Autodesk Inventor part; units mm, degrees
ref_plane "YZ Plane" through (0, 0, 0) normal (1, 0, 0) x (0, 1, 0)
ref_plane "XZ Plane" through (0, 0, 0) normal (0, 1, 0) x (-1, 0, 0)
ref_plane "XY Plane" through (0, 0, 0) normal (0, 0, 1) x (1, 0, 0)
sketch "Skizze_1" plane through (0, 0, 0) normal (1, 0, 0) x (0, 0, 1)
  line L0 (0, 0) -> (-19.95, 0)
  line L1 (-19.95, 0) -> (-19.95, -4)
  line L2 (-19.95, -4) -> (-14, -4)
  line L3 (-14, -4) -> (-14, -10.5)
  line L4 (-14, -10.5) -> (-15.5, -12)
  line L5 (-15.5, -12) -> (-34.5, -12)
  line L6 (-34.5, -12) -> (-36, -10.5)
  line L7 (-36, -10.5) -> (-36, -4)
  line L8 (-36, -4) -> (-30.05, -4)
  line L9 (-30.05, -4) -> (-30.05, 0)
  line L10 (-30.05, 0) -> (-50, 0)
  line L11 (-50, 0) -> (-50, -19.95)
  line L12 (-50, -19.95) -> (-46, -19.95)
  line L13 (-46, -19.95) -> (-46, -14)
  line L14 (-46, -14) -> (-39.5, -14)
  line L15 (-39.5, -14) -> (-38, -15.5)
  line L16 (-38, -15.5) -> (-38, -34.5)
  line L17 (-38, -34.5) -> (-39.5, -36)
  line L18 (-39.5, -36) -> (-46, -36)
  line L19 (-46, -36) -> (-46, -30.05)
  line L20 (-46, -30.05) -> (-50, -30.05)
  line L21 (-50, -30.05) -> (-50, -50)
  line L22 (-50, -50) -> (-30.05, -50)
  line L23 (-30.05, -50) -> (-30.05, -46)
  line L24 (-30.05, -46) -> (-36, -46)
  line L25 (-36, -46) -> (-36, -39.5)
  line L26 (-36, -39.5) -> (-34.5, -38)
  line L27 (-34.5, -38) -> (-15.5, -38)
  line L28 (-15.5, -38) -> (-14, -39.5)
  line L29 (-14, -39.5) -> (-14, -46)
  line L30 (-14, -46) -> (-19.95, -46)
  line L31 (-19.95, -46) -> (-19.95, -50)
  line L32 (-19.95, -50) -> (0, -50)
  line L33 (0, -50) -> (0, -30.05)
  line L34 (0, -30.05) -> (-4, -30.05)
  line L35 (-4, -30.05) -> (-4, -36)
  line L36 (-4, -36) -> (-10.5, -36)
  line L37 (-10.5, -36) -> (-12, -34.5)
  line L38 (-12, -34.5) -> (-12, -15.5)
  line L39 (-12, -15.5) -> (-10.5, -14)
  line L40 (-10.5, -14) -> (-4, -14)
  line L41 (-4, -14) -> (-4, -19.95)
  line L42 (-4, -19.95) -> (0, -19.95)
  line L43 (0, -19.95) -> (0, 0)
  circle A0 centre (-42.5, -42.5) radius 3.5
  circle A1 centre (-42.5, -7.5) radius 3.5
  line L44 (-14.95, -35.05) -> (-14.95, -14.95)
  line L45 (-14.95, -14.95) -> (-35.05, -14.95)
  line L46 (-35.05, -14.95) -> (-35.05, -35.05)
  line L47 (-35.05, -35.05) -> (-14.95, -35.05)
  circle A2 centre (-7.5, -42.5) radius 3.5
  circle A3 centre (-7.5, -7.5) radius 3.5
extrude "MK, 50MM" add sketch "Skizze_1" along normal blind 100
properties part number "BAR, EXTRUDED ALUM, 50MMX50MM, MK, 2000 SERIES" material "Aluminum, 6061-T6"
Can you work these out from the model? Positions are in its coordinate system, mm. A direction names the side the tool comes from. Round coordinates to 2 decimals unless told otherwise and drop trailing zeros. Loops run counter-clockwise (first coordinate to the right, second up) from the corner with the lowest first, then second, coordinate; pieces in that order, holes last. Notation, with made-up numbers: M 2.5,-11.75 L 38.5,-11.75 A10 cw 38.5,-2.75 Z; hole C 5.5,-23.75 d8. An arc over 180 degrees is marked long. Answer as a JSON object with one key per item and string values. Group by question number.
Q1. Imagine slicing it at B-B, the plane y = 42.5. Please give me the cut outline in (x, z).
Q2. Imagine slicing it at C-C, the plane z = -18. Please give me the cut outline in (x, y).
Q3. Please list where these lines run through material, in increasing order: L1, parallel to Z at x = 46, y = 42.5; L2, parallel to Y at x = 79, z = -42.5; L3, parallel to Z at x = 32.5, y = 16.
Q4. Will these pins go through, and if not, where does the flat tip stop? pin 1 (1.5 mm diameter, centred on y = 5.5, z = -35.5, fed in from +X); pin 2 (3 mm diameter, centred on x = 33, z = -28.5, fed in from +Y).
Q5. We'd pull the mould along Y, two halves only. Please class faces 5 (the flat face through (100, 14, -25)), 6 (the flat face through (49, 4, -17)), 7 (the flat face through (49, 30.05, -2)), 8 (the flat face through (49, 50, -40)): +Y half, -Y half, draft (parallel to the pull), parting line (faces both ways), or undercut.
Q6. Imagine slicing it at D-D, the plane y = 29. Please give me the cut outline in (x, z).
Q7. Imagine slicing it at A-A, the plane z = -29. Please give me the cut outline in (x, y).
Q8. On a 3-axis mill with a long thin cutter (end or side, diameter ignored), from which of +Z, -Z, +X, -X, +Y, -Y can I reach the whole of each face in a straight line? I mean faces 1 (the flat face through (49, 2, -30.05)), 2 (the flat face through (0, 14, -25)), 3 (the flat face through (49, 25, -35.05)), 4 (the flat face through (49, 30.05, -48)). Say none if no direction works.
Findings:
{
 "1": {"outline": "M 0,-50 L 100,-50 L 100,-46 L 0,-46 Z; M 0,-39 L 100,-39 L 100,-36 L 0,-36 Z; M 0,-14 L 100,-14 L 100,-11 L 0,-11 Z; M 0,-4 L 100,-4 L 100,0 L 0,0 Z"},
 "2": {"outline": "M 0,0 L 100,0 L 100,4 L 0,4 Z; M 0,12 L 100,12 L 100,14.95 L 0,14.95 Z; M 0,35.05 L 100,35.05 L 100,38 L 0,38 Z; M 0,46 L 100,46 L 100,50 L 0,50 Z"},
 "3": {"L1": "z = -50 to -46, -39 to -36, -14 to -11, -4 to 0", "L2": "y = 0 to 4, 11 to 14, 36 to 39, 46 to 50", "L3": "z = -50 to -46, -38 to -35.05, -14.95 to -12, -4 to 0"},
 "4": {"pin 1": "stops at x = 100", "pin 2": "stops at y = 38"},
 "5": {"face 5": "draft", "face 6": "undercut", "face 7": "undercut", "face 8": "+Y half"},
 "6": {"outline": "M 0,-38 L 100,-38 L 100,-35.05 L 0,-35.05 Z; M 0,-14.95 L 100,-14.95 L 100,-12 L 0,-12 Z"},
 "7": {"outline": "M 0,12 L 100,12 L 100,14.95 L 0,14.95 Z; M 0,35.05 L 100,35.05 L 100,38 L 0,38 Z"},
 "8": {"face 1": "+X, -X, -Y", "face 2": "+Z, -Z, -X, +Y, -Y", "face 3": "+X, -X", "face 4": "-Z, +X, -X"}
}
